For this review, use the dimensioned drawing (mm, ordinates from the lowest corner) and the shaded views. Round coordinates to 2 decimals unless told otherwise and drop trailing zeros. Order: outer loops, then holes, each group sorted by start corner. A loop starts at its lowest first (then second) coordinate and runs counter-clockwise, first axis right, second up. Notation, with made-up numbers: M 10,63.5 L 39,63.5 A34 ccw 39,97.5 Z; hole C -7,-16.75 d8. An arc over 180 degrees is marked long. Answer as CSV lines item,"result". Start each with the question number.
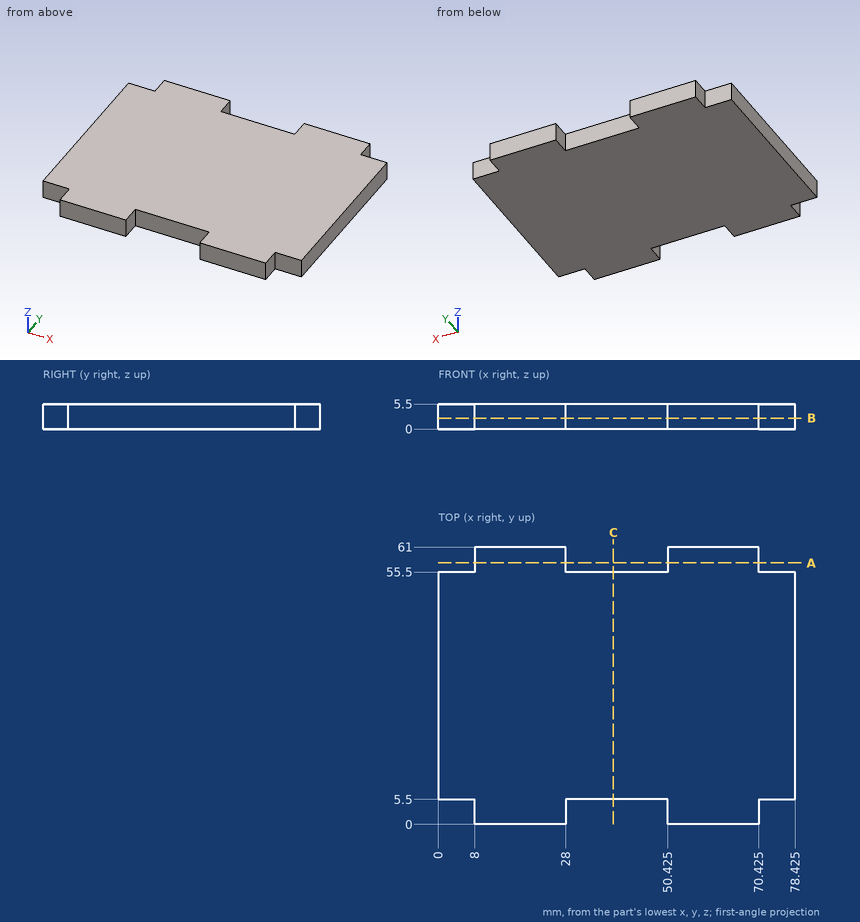
Item 1: Wall thickness on probe 1 along X at (y, z) = (57, 3.6) (3 decimals); probe 2 along Y at (x, z) = (37, 0.2): over which ranges is each line inside the solid? List them lowest first. Write a range as [from, to].
Item 2: For pin 1 (1.6 mm diameter, centred on y = 2, z = 4, fed in from +X) (3 decimals); pin 2 (10 mm diameter, centred on x = 59.5, y = 16, fed in from -Z); pin 3 (1.6 mm diameter, centred on x = 74, z = 2.5, fed in from +Y); pin 4 (1.6 mm diameter, centred on x = 73.5, z = 2, fed in from -Y), all flat-tipped, find the tip position at first contact; note any pin that passes through.
Item 3: Consider section C-C (x = 38.5). State the section outline as (y, z) points.
Item 4: Consider section B-B (z = 2.4). State the section outline as (x, y) points (3 decimals), and give its area (3 significant figures).
Item 5: Consider section A-A (y = 57.5). State the section outline as (x, z) points (3 decimals).
Reported:
1,probe 1,"x = [8, 28], [50.425, 70.425]"
1,probe 2,"y = [5.5, 55.5]"
2,pin 1,"stops at x = 70.425"
2,pin 2,"stops at z = 0"
2,pin 3,"stops at y = 55.5"
2,pin 4,"stops at y = 5.5"
3,outline,"M 5.5,0 L 55.5,0 L 55.5,5.5 L 5.5,5.5 Z"
4,outline,"M 0,5.5 L 8,5.5 L 8,0 L 28,0 L 28,5.5 L 50.425,5.5 L 50.425,0 L 70.425,0 L 70.425,5.5 L 78.425,5.5 L 78.425,55.5 L 70.425,55.5 L 70.425,61 L 50.425,61 L 50.425,55.5 L 28,55.5 L 28,61 L 8,61 L 8,55.5 L 0,55.5 Z"
4,area,"4,360 mm²"
5,outline,"M 8,0 L 28,0 L 28,5.5 L 8,5.5 Z; M 50.425,0 L 70.425,0 L 70.425,5.5 L 50.425,5.5 Z"
